from build123d import *

# Parameters (mm, degrees)
SKETCH1_R           = 101.6
BOSS_EXTRUDE1_DEPTH = 9.525
SKETCH2_R           = 4.7625
SKETCH2_R_2         = 3.175
CUT_EXTRUDE1_DEPTH  = 22.86
SKETCH3_R           = 4.7625
CUT_EXTRUDE2_DEPTH  = 144.999463975
FILLET1_R           = 2.54
FILLET3_R           = 2.54
SKETCH4_R           = 5.715
CUT_EXTRUDE3_DEPTH  = 17.78


with BuildPart() as part:
    # Sketch1 → Boss-Extrude1 (new body)
    with BuildSketch(Plane(origin=(0, 0, 0), x_dir=(1, 0, 0), z_dir=(0, 1, 0))):
        with Locations(Location((0, 0, 0), (0, 0, 90))):
            Circle(SKETCH1_R)
    extrude(amount=BOSS_EXTRUDE1_DEPTH)

    # Sketch2 → Cut-Extrude1 (cut)
    with BuildSketch(Plane(origin=(0, 9.525, 0), x_dir=(1, 0, 0), z_dir=(0, 1, 0))):
        with BuildLine():
            Line((-9.955759688, 26.595729902), (-15.303128109, -23.922045692))
            ThreePointArc((-15.303128109, -23.922045692), (-4.010526316, -37.888331696), (9.955759688, -26.595729902))
            Line((9.955759688, -26.595729902), (15.303128109, 23.922045692))
            ThreePointArc((15.303128109, 23.922045692), (4.010526316, 37.888331696), (-9.955759688, 26.595729902))
        make_face()
        with Locations(Location((34.817520913, 15.470948176, 0), (0, 0, 270))):
            Circle(SKETCH2_R)
        with Locations(Location((-34.817520913, -15.470948176, 0), (0, 0, 270))):
            Circle(SKETCH2_R)
        with BuildLine():
            Line((-30.765292524, 38.093536125), (-87.237043764, 79.186441231))
            Line((-87.237043764, 79.186441231), (-104.485964967, 60.325))
            Line((-104.485964967, 60.325), (-45.710214871, 17.555539727))
            ThreePointArc((-45.710214871, 17.555539727), (-27.968755498, 20.352076753), (-30.765292524, 38.093536125))
        make_face()
        with Locations(Location((5.646300897, 53.341856998, 0), (0, 0, 270))):
            Circle(SKETCH2_R_2)
        with Locations(Location((31.560768513, 43.372252797, 0), (0, 0, 270))):
            Circle(SKETCH2_R_2)
        with Locations(Location((-53.341856998, 5.646300897, 0), (0, 0, 270))):
            Circle(SKETCH2_R_2)
        with Locations(Location((43.372252797, -31.560768513, 0), (0, 0, 270))):
            Circle(SKETCH2_R_2)
        with Locations(Location((-49.018553694, -21.781088485, 0), (0, 0, 270))):
            Circle(SKETCH2_R_2)
        with Locations(Location((21.781088485, -49.018553694, 0), (0, 0, 270))):
            Circle(SKETCH2_R_2)
    extrude(amount=-CUT_EXTRUDE1_DEPTH, mode=Mode.SUBTRACT)

    # Sketch3 → Cut-Extrude2 (cut, through all)
    with BuildSketch(Plane(origin=(0, 9.525, 0), x_dir=(1, 0, 0), z_dir=(0, 1, 0))):
        with BuildLine():
            Line((61.173834056, -33.71623536), (83.418864622, -45.976684582))
            ThreePointArc((83.418864622, -45.976684582), (95.231198209, 1.892455481), (81.526409141, 49.254513627))
            Line((81.526409141, 49.254513627), (59.78603337, 36.119976659))
            ThreePointArc((59.78603337, 36.119976659), (69.83621202, 1.387800686), (61.173834056, -33.71623536))
        make_face()
        with BuildLine():
            ThreePointArc((50.898077232, -47.837310063), (20.160372855, -66.87736438), (-15.979287148, -67.997682918))
            Line((-15.979287148, -67.997682918), (-21.78993702, -92.72411307))
            ThreePointArc((-21.78993702, -92.72411307), (27.491417529, -91.196405972), (69.406468953, -65.232695541))
            Line((69.406468953, -65.232695541), (50.898077232, -47.837310063))
        make_face()
        with BuildLine():
            ThreePointArc((-59.78603337, -36.119976659), (-69.466812234, -7.306469604), (-65.992729528, 22.890656378))
            Line((-65.992729528, 22.890656378), (-87.200441174, 38.322911673))
            ThreePointArc((-87.200441174, 38.322911673), (-95.050717303, -6.15821729), (-81.526409141, -49.254513627))
            Line((-81.526409141, -49.254513627), (-59.78603337, -36.119976659))
        make_face()
        with BuildLine():
            Line((-63.288565419, 71.183705911), (-42.080853774, 55.751450615))
            ThreePointArc((-42.080853774, 55.751450615), (-14.415807175, 68.34622889), (15.979287148, 67.997682918))
            Line((15.979287148, 67.997682918), (21.78993702, 92.72411307))
            ThreePointArc((21.78993702, 92.72411307), (-23.37800943, 92.33651052), (-63.288565419, 71.183705911))
        make_face()
        with Locations(Location((42.966651746, 59.046739645, 0), (0, 0, 270))):
            Circle(SKETCH3_R)
        with Locations(Location((-42.966651746, -59.046739645, 0), (0, 0, 270))):
            Circle(SKETCH3_R)
    extrude(amount=-CUT_EXTRUDE2_DEPTH, mode=Mode.SUBTRACT)

    # Fillet1
    fillet1_edges = [part.edges().sort_by_distance(p)[0] for p in [
        (-74.035185173, 4.7625, -69.579820037),
        (-88.980107519, 4.7625, -49.041823639),
    ]]
    fillet(fillet1_edges, radius=FILLET1_R)

    # Fillet3
    fillet3_edges = [part.edges().sort_by_distance(p)[0] for p in [
        (15.979287148, 4.7625, -67.997682918),
        (-42.080853774, 4.7625, -55.751450615),
        (-63.288565419, 4.7625, -71.183705911),
        (21.78993702, 4.7625, -92.72411307),
        (59.78603337, 4.7625, -36.119976659),
        (81.526409141, 4.7625, -49.254513627),
        (83.418864622, 4.7625, 45.976684582),
        (61.173834056, 4.7625, 33.71623536),
        (-15.979287148, 4.7625, 67.997682918),
        (50.898077232, 4.7625, 47.837310063),
        (69.406468953, 4.7625, 65.232695541),
        (-21.78993702, 4.7625, 92.72411307),
        (-59.78603337, 4.7625, 36.119976659),
        (-81.526409141, 4.7625, 49.254513627),
        (-87.200441174, 4.7625, -38.322911673),
        (-65.992729528, 4.7625, -22.890656378),
    ]]
    fillet(fillet3_edges, radius=FILLET3_R)

    # Sketch4 → Cut-Extrude3 (cut)
    with BuildSketch(Plane(origin=(0, 9.525, 0), x_dir=(1, 0, 0), z_dir=(0, 1, 0))):
        with Locations(Location((42.966651746, 59.046739645, 0), (0, 0, 270))):
            Circle(SKETCH4_R)
        with Locations(Location((-42.966651746, -59.046739645, 0), (0, 0, 270))):
            Circle(SKETCH4_R)
        with Locations(Location((-34.817520913, -15.470948176, 0), (0, 0, 270))):
            Circle(SKETCH4_R)
        with Locations(Location((34.817520913, 15.470948176, 0), (0, 0, 270))):
            Circle(SKETCH4_R)
    extrude(amount=-CUT_EXTRUDE3_DEPTH, mode=Mode.SUBTRACT)


solid = part.part
Work out the finished part from the listing and answer in its coordinate system (mm). A direction names the side the tool comes from. Give positions to 0.01 mm unless a question says otherwise; leave off trailing zeros. Order: outer loops, then holes, each group sorted by start corner. A loop starts at its lowest first (then second) coordinate and runs counter-clockwise, first axis right, second up. Notation, with made-up numbers: (55.5, -38) -> (80.5, -38) arc R9 ccw to (80.5, -23) -> close; hole circle Ø8 at (4.25, 56.25). An arc over 180 degrees is marked (long way). Answer as a JSON object with one key per item and string values. Group by question number.
1. The mould has two halves that part along X. Classify faces 3 (the cylindrical face through (79.58, 4.7, 63.16)), 4 (the flat face through (21, 0, 1)), 5 (the cylindrical face through (-22.486, 4.829, -92.558)): released by +X, released by -X, zero draft, split by the parting line, or undercut.
2. Section C-C on y = 6.5 is taken. Count the separate pieces of the cut face and the enclosed holes in it, plus the area to 3 significant figures.
3. Section B-B on z = 0 is taken. Determine the outline of the cut face in (x, y) (3 decimals), plus the area to 3 significant figures.
4. Consider line 1 along X through (y, z) = (6.5, 33); line 2 along X through (y, z) = (3.25, 43); line 3 along Z through (x, y) = (61, 1.25). Determine where each line is inside the solid, lowest interval first. Write a range as [from, to].
5. A tool of negligible diameter and unlimited length cuts with its end or side. For faces 1 (the flat face through (12.592, 4.829, 1.69)), 2 (the flat face through (21, 9.525, 1)), from which of +Z, -Z, +X, -X, +Y, -Y can it reach the whole face along a straight path? Write none if from no direction.
6. Flat-ended cylindrical pins translate along their axes: pin 1 Ø3 at (y, z) = (4.5, -58) entering from +X; pin 2 Ø4 at (x, y) = (18.5, 4) entering from +Z; pin 3 Ø4 at (y, z) = (3.5, -62.5) entering from -X. Find the tip coordinate at first contact, or state that the pin passes through.
7. Section A-A on x = 0 is taken. Determine the outline of the cut face in (y, z) (3 decimals).
Result sheet:
{
 "1": {"face 3": "split by the parting line", "face 4": "zero draft", "face 5": "undercut"},
 "2": {"separate pieces": "1", "enclosed holes": "15", "area": "20,200 mm^2"},
 "3": {"outline": "(-101.6, 0) -> (-95.25, 0) -> (-95.25, 9.525) -> (-101.6, 9.525) -> close; (-69.85, 0) -> (-12.771, 0) -> (-12.771, 9.525) -> (-69.85, 9.525) -> close; (12.771, 0) -> (69.85, 0) -> (69.85, 9.525) -> (12.771, 9.525) -> close; (95.25, 0) -> (101.6, 0) -> (101.6, 9.525) -> (95.25, 9.525) -> close", "area": "1,210 mm^2"},
 "4": {"line 1": "x = [-96.09, -89.35], [-61.56, -12.74], [7.39, 40.54], [46.2, 62.06], [89.35, 96.09]", "line 2": "x = [-92.05, -84.99], [-71.17, 78.02], [84.99, 92.05]", "line 3": "z = [-81.25, -36.44], [-34.03, 57.33], [73.15, 81.25]"},
 "5": {"face 1": "+Y, -Y", "face 2": "+Z, -Z, +X, -X, +Y"},
 "6": {"pin 1": "stops at x = 84.44", "pin 2": "stops at z = 100.25", "pin 3": "stops at x = -67.05"},
 "7": {"outline": "(0, -101.6) -> (9.525, -101.6) -> (9.525, -95.25) -> (0, -95.25) -> close; (0, -69.85) -> (9.525, -69.85) -> (9.525, -37.674) -> (0, -37.674) -> close; (0, 37.674) -> (9.525, 37.674) -> (9.525, 69.85) -> (0, 69.85) -> close; (0, 95.25) -> (9.525, 95.25) -> (9.525, 101.6) -> (0, 101.6) -> close"}
}
